```python
from build123d import *

# Parameters (mm, degrees)
EXTRUDE_THIN1_DEPTH = 269.875
FILLET1_R           = 0.889


with BuildPart() as part:
    # Sketch1 → Extrude-Thin1 (new body)
    with BuildSketch(Plane.XY):
        with BuildLine():
            Line((10.31875, 0), (13.49375, 0))
            Line((13.49375, 0), (13.49375, 3.96875))
            Line((13.49375, 3.96875), (11.1125, 3.96875))
            Line((11.1125, 3.96875), (11.1125, 5.55625))
            ThreePointArc((11.1125, 5.55625), (9.428701977, 6.253701977), (8.73125, 7.9375))
            ThreePointArc((8.73125, 7.9375), (7.336346045, 11.305096045), (3.96875, 12.7))
            Line((3.96875, 12.7), (3.96875, 15.08125))
            Line((3.96875, 15.08125), (-3.96875, 15.08125))
            Line((-3.96875, 15.08125), (-3.96875, 12.7))
            ThreePointArc((-3.96875, 12.7), (-7.336346045, 11.305096045), (-8.73125, 7.9375))
            ThreePointArc((-8.73125, 7.9375), (-9.428701977, 6.253701977), (-11.1125, 5.55625))
            Line((-11.1125, 5.55625), (-11.1125, 3.96875))
            Line((-11.1125, 3.96875), (-13.49375, 3.96875))
            Line((-13.49375, 3.96875), (-13.49375, 0))
            Line((-13.49375, 0), (-10.31875, 0))
            Line((-10.31875, 0), (-10.31875, 0.889))
            Line((-10.31875, 0.889), (-12.60475, 0.889))
            Line((-12.60475, 0.889), (-12.60475, 3.07975))
            Line((-12.60475, 3.07975), (-10.2235, 3.07975))
            Line((-10.2235, 3.07975), (-10.2235, 4.790403868))
            ThreePointArc((-10.2235, 4.790403868), (-8.504647693, 5.96426879), (-7.84225, 7.9375))
            ThreePointArc((-7.84225, 7.9375), (-6.372960967, 10.974566327), (-3.07975, 11.707603613))
            Line((-3.07975, 11.707603613), (-3.07975, 14.19225))
            Line((-3.07975, 14.19225), (3.07975, 14.19225))
            Line((3.07975, 14.19225), (3.07975, 11.707603613))
            ThreePointArc((3.07975, 11.707603613), (6.372960967, 10.974566327), (7.84225, 7.9375))
            ThreePointArc((7.84225, 7.9375), (8.504647693, 5.96426879), (10.2235, 4.790403868))
            Line((10.2235, 4.790403868), (10.2235, 3.07975))
            Line((10.2235, 3.07975), (12.60475, 3.07975))
            Line((12.60475, 3.07975), (12.60475, 0.889))
            Line((12.60475, 0.889), (10.31875, 0.889))
            Line((10.31875, 0.889), (10.31875, 0))
        make_face()
    extrude(amount=-EXTRUDE_THIN1_DEPTH)

    # Fillet1
    fillet1_edges = [part.edges().sort_by_distance(p)[0] for p in [
        (-13.49375, 0, -134.9375),
        (-13.49375, 3.96875, -134.9375),
        (-11.1125, 5.55625, -134.9375),
        (-3.96875, 15.08125, -134.9375),
        (3.96875, 15.08125, -134.9375),
        (11.1125, 5.55625, -134.9375),
        (13.49375, 3.96875, -134.9375),
        (13.49375, 0, -134.9375),
        (10.2235, 3.07975, -134.9375),
        (3.07975, 11.707603613, -134.9375),
        (-3.07975, 11.707603613, -134.9375),
        (-10.2235, 3.07975, -134.9375),
    ]]
    fillet(fillet1_edges, radius=FILLET1_R)


solid = part.part
```
Model file for the job. Use its own axes, mm. Coordinates: 2 decimals unless noted, no trailing zeros. One line per item, written item: value. Start each with the question number.
1. Flat gauge pins, fed straight in: pin 1 (0.7 mm diameter, centred on x = -11.5, z = -168.5, fed in from +Y); pin 2 (2.5 mm diameter, centred on x = -11, z = -82, fed in from +Y); pin 3 (3 mm diameter, centred on y = 11.5, z = -216, fed in from +X). Where does each tip first touch, or does it go through?
2. Mould opens along X. For faces 1 (the cylindrical face through (-7.3, 11.34, -133.05)), 2 (the flat face through (0, 14.192, -133)), 3 (the flat face through (0, 15.081, -133)) say: released by +X, released by -X, zero draft, split by the parting line, or undercut.
3. Probe line 1 (X direction, y = 13, z = -214); line 2 (X direction, y = 2.25, z = -28); line 3 (Y direction, x = -4.25, z = -106.5). List the from-to ranges inside material, lowest first. Write a range as from..to.
Answers below:
1. pin 1: stops at y = 3.97
1. pin 2: stops at y = 5.98
1. pin 3: stops at x = 8.26
2. face 1: released by -X
2. face 2: undercut
2. face 3: zero draft
3. line 1: x = -3.97..-3.08, 3.08..3.97
3. line 2: x = -13.49..-12.6, 12.6..13.49
3. line 3: y = 11.8..12.69
